For this review, take the finished solid that the model builds, in its own axes (mm). A direction names the side the tool comes from. Round coordinates to 2 decimals unless told otherwise and drop trailing zeros. Write each loop counter-clockwise with the first axis right and the second up, starting at its lowest first coordinate (ties: lowest second). Pieces come first, ordered by that corner, then holes.
from build123d import *

# Parameters (mm, degrees)
F1_DEPTH      = 1400
F3_DEPTH      = 35
F3_DEPTH_BACK = 35
F6_DEPTH      = 2


with BuildPart() as f1:
    # F0 (on Top) → F1 (new body)
    with BuildSketch(Plane.XY):
        with BuildLine():
            ThreePointArc((-35, -33), (-34.4142135624, -34.4142135624), (-33, -35))
            Line((-33, -35), (33, -35))
            ThreePointArc((33, -35), (34.4142135624, -34.4142135624), (35, -33))
            Line((35, -33), (35, 33))
            ThreePointArc((35, 33), (34.4142135624, 34.4142135624), (33, 35))
            Line((33, 35), (-33, 35))
            ThreePointArc((-33, 35), (-34.4142135624, 34.4142135624), (-35, 33))
            Line((-35, 33), (-35, -33))
        make_face()
        with BuildLine():
            Line((32, -33), (-32, -33))
            ThreePointArc((-32, -33), (-32.7071067812, -32.7071067812), (-33, -32))
            Line((-33, -32), (-33, 32))
            ThreePointArc((-33, 32), (-32.7071067812, 32.7071067812), (-32, 33))
            Line((-32, 33), (32, 33))
            ThreePointArc((32, 33), (32.7071067812, 32.7071067812), (33, 32))
            Line((33, 32), (33, -32))
            ThreePointArc((33, -32), (32.7071067812, -32.7071067812), (32, -33))
        make_face(mode=Mode.SUBTRACT)
    extrude(amount=F1_DEPTH)

    # F2 (on Front) → F3 (cut, two sides)
    with BuildSketch(Plane.XZ) as f3_sk:
        Polygon((-35, 1400), (35, 1380), (35, 1400), align=None)
    extrude(amount=-F3_DEPTH, mode=Mode.SUBTRACT)
    extrude(f3_sk.sketch, amount=F3_DEPTH_BACK, mode=Mode.SUBTRACT)

    # F5 (on offset) → F6 (join)
    with BuildSketch(Plane(origin=(367.1698113208, 0, 1285.0943396226), x_dir=(0.9615239476, 0, -0.2747211279), z_dir=(0.2747211279, 0, 0.9615239476))):
        with BuildLine():
            Line((-341.461818331, 40), (-422.2629172238, 40))
            ThreePointArc((-422.2629172238, 40), (-422.9700240049, 39.7071067812), (-423.2629172238, 39))
            Line((-423.2629172238, 39), (-423.2629172238, -39))
            ThreePointArc((-423.2629172238, -39), (-422.9700240049, -39.7071067812), (-422.2629172238, -40))
            Line((-422.2629172238, -40), (-341.461818331, -40))
            ThreePointArc((-341.461818331, -40), (-340.7547115498, -39.7071067812), (-340.461818331, -39))
            Line((-340.461818331, -39), (-340.461818331, 39))
            ThreePointArc((-340.461818331, 39), (-340.7547115498, 39.7071067812), (-341.461818331, 40))
        make_face()
    extrude(amount=F6_DEPTH)


solid = f1.part
(1) We need section B-B, the plane y = -7. Give the boundary of the cut face in (x, z), and give its area (3 significant figures).
Geometry check:
outline: (-39.81, 1401.37) - (-35, 1400) - (-35, 0) - (-33, 0) - (-33, 1399.43) - (33, 1380.57) - (33, 0) - (35, 0) - (35, 1380) - (39.81, 1378.63) - (40.36, 1380.55) - (-39.26, 1403.3) - close
area: 5,730 mm2
(2) For pin 1 Ø2 at (y, z) = (8, 271) entering from -X; pin 2 Ø1.5 at (x, y) = (-24.5, -27.5) entering from +Z; pin 3 Ø19 at (x, z) = (-5, 509.5) entering from -Y, all flat-tipped, find the tip position at first contact; note any pin that passes through.
Geometry check:
pin 1: stops at x = -35
pin 2: stops at z = 1399.29
pin 3: stops at y = -35
(3) We need section A-A, the plane z = 689. Give the boundary of the cut face in (x, y).
Geometry check:
outline: (-35, -33) arc R2 ccw to (-33, -35) - (33, -35) arc R2 ccw to (35, -33) - (35, 33) arc R2 ccw to (33, 35) - (-33, 35) arc R2 ccw to (-35, 33) - close; hole (-33, -32) arc R1 ccw to (-32, -33) - (32, -33) arc R1 ccw to (33, -32) - (33, 32) arc R1 ccw to (32, 33) - (-32, 33) arc R1 ccw to (-33, 32) - close
(4) For faces 4 (the face through (0, -40, 1391)), 5 (the face through (-33, 0, 690)), list the 3-axis set-ups (+Z, -Z, +X, -X, +Y, -Y) from which the entire face can be reached by the end or side of a thin tool; tool diameter is ignored.
Geometry check:
face 4: +Z, -Z, +X, -X, -Y
face 5: -Z
(5) We need section C-C, the plane x = 1.5. Give the boundary of the cut face in (y, z), and give its area (3 significant figures).
Geometry check:
outline: (-40, 1389.57) - (-35, 1389.57) - (-35, 0) - (-33, 0) - (-33, 1389.57) - (33, 1389.57) - (33, 0) - (35, 0) - (35, 1389.57) - (40, 1389.57) - (40, 1391.65) - (-40, 1391.65) - close
area: 5,720 mm2
(6) For line 1 along Y through (x, z) = (18.5, 846); line 2 along Y through (x, z) = (-33.5, 1082), list the stretches that pass through material, from the lowest coordinate up.
Geometry check:
line 1: y = -35 to -33, 33 to 35
line 2: y = -34.94 to 34.94
(7) Mouldability with a two-part tool opening along Y and no side actions: class faces 1 (the face through (0, 35, 690)), 2 (the face through (0, 33, 690)), 3 (the face through (-35, 0, 690)) as pulls with the +Y half, pulls with the -Y half, needs draft (parallel to the pull), parting line crosses it, or undercut.
Geometry check:
face 1: pulls with the +Y half
face 2: undercut
face 3: needs draft
